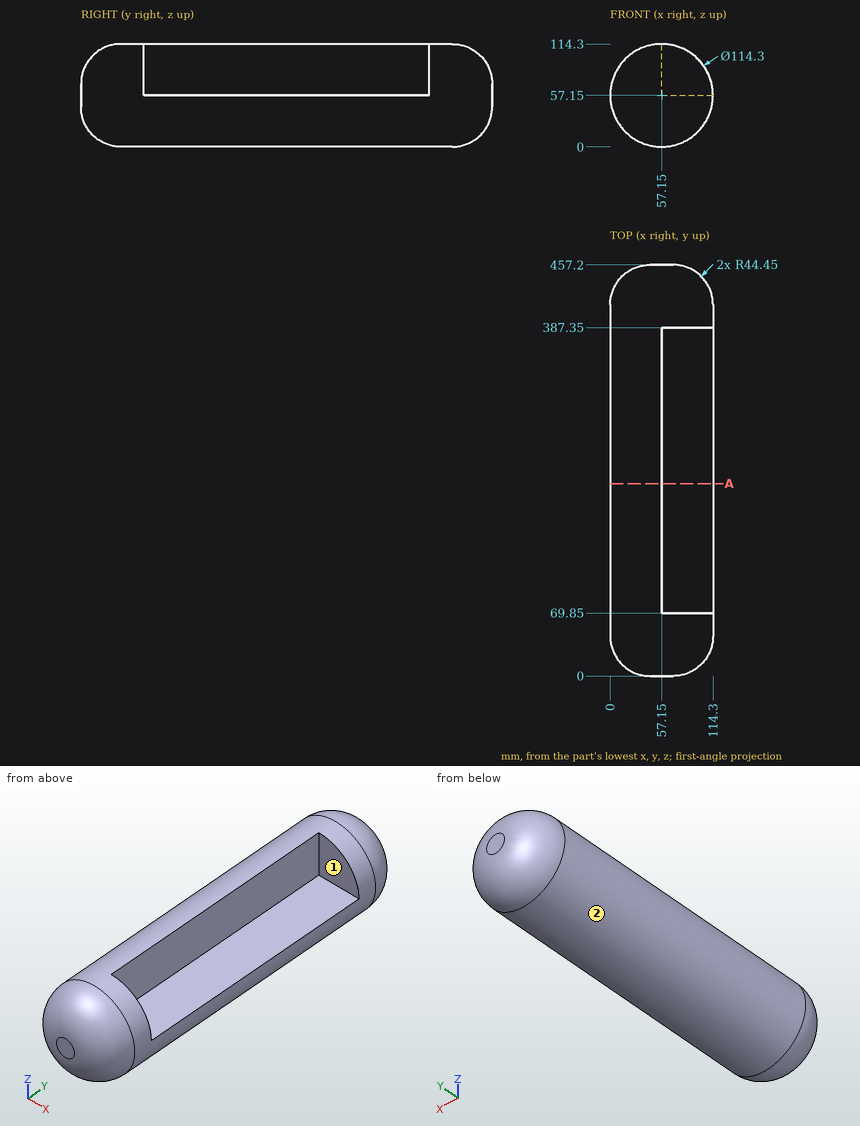
Part print with two shaded views. Sizes in mm from the minimum x, y, z corner. A direction names the side the tool comes from. Round coordinates to 2 decimals unless told otherwise and drop trailing zeros. Loops run counter-clockwise (first coordinate to the right, second up) from the corner with the lowest first, then second, coordinate; pieces in that order, holes last. Notation, with made-up numbers: (-12, 50.5) - (14, 50.5) arc R20 ccw to (14, 86.5) - close; hole circle Ø3 at (73, 7.5). An arc over 180 degrees is marked (long way). Put each result on its own line as item: value.
1. 3-axis set-ups, long thin cutter, end or side, ignore diameter. For the marked faces 1 and 2: which of +Z, -Z, +X, -X, +Y, -Y reach the whole face in a straight line?
Geometry check:
face 1: +Z, +X
face 2: +Y, -Y
2. Slice it at A-A on y = 214. List the corners of the cut face in (x, z), and give its area (3 significant figures).
Geometry check:
outline: (57.15, 57.15) - (57.15, 114.3) arc R57.15 ccw (long way) to (114.3, 57.15) - close
area: 7,700 mm²
3. Pin check, flat tips, straight feed: P1, Ø6, axis at x = 90.5, z = 99, coming from the +Y side; P2, Ø6, axis at y = 182.5, z = 19, coming from the -X side; P3, Ø17, axis at y = 174.5, z = 84.5, coming from the +X side. Stop position of each tip, or through.
Geometry check:
P1: y = 436.12
P2: x = 12.09
P3: x = 57.15
4. Wall check: line 1 (Y direction, x = 60, z = 60); line 2 (Y direction, x = 65.5, z = 95.5); line 3 (X direction, y = 90, z = 59.5). Give the ranges that are in metal, low to high.
Geometry check:
line 1: 0 to 69.85, 387.35 to 457.2
line 2: 8.8 to 69.85, 387.35 to 448.4
line 3: 0.05 to 57.15
